For this review, take the finished solid that the model builds, in its own axes (mm). A direction names the side the tool comes from. Coordinates: 2 decimals unless noted, no trailing zeros. Write each loop counter-clockwise with the first axis right and the second up, starting at its lowest first coordinate (ties: lowest second). Pieces come first, ordered by that corner, then holes.
Autodesk Inventor part; units mm, degrees
ref_plane "YZ Plane" through (0, 0, 0) normal (1, 0, 0) x (0, 1, 0)
ref_plane "XZ Plane" through (0, 0, 0) normal (0, 1, 0) x (-1, 0, 0)
ref_plane "XY Plane" through (0, 0, 0) normal (0, 0, 1) x (1, 0, 0)
sketch "Sketch1" plane through (0, 0, 0) normal (0, 0, 1) x (1, 0, 0)
  line L0 (0, 0) -> (25.4, 0)
  line L1 (25.4, 0) -> (25.4, 25.4)
  line L2 (25.4, 25.4) -> (0, 25.4)
  line L3 (0, 25.4) -> (0, 0)
  line L4 (3.175, 22.225) -> (22.225, 22.225)
  line L5 (22.225, 22.225) -> (22.225, 3.175)
  line L6 (22.225, 3.175) -> (3.175, 3.175)
  line L7 (3.175, 3.175) -> (3.175, 22.225)
  dimension "d0" = 25.4
  dimension "d1" = 25.4
  dimension "d2" = 3.175
extrude "Extrusion1" add sketch "Sketch1" along normal blind 101.6
sketch "Sketch2" plane through (25.4, 0, 0) normal (1, 0, 0) x (0, 0, -1)
  line L0 (0, 0) -> (0, 25.4)
  line L1 (-101.6, 0) -> (-101.6, 25.4)
  line L2 (0, 0) -> (-101.6, 0)
  circle A0 centre (-88.9, 12.7) radius 2.0701
  circle A1 centre (-76.2, 12.7) radius 2.0701
  circle A2 centre (-12.7, 12.7) radius 3.3782
  dimension "d5" = 4.1402
  dimension "d6" = 12.7
  dimension "d7" = 12.7
  dimension "d10" = 12.7
  dimension "d15" = 6.7564
  dimension "d16" = 12.7
  dimension "d17" = 12.7
extrude "Extrusion2" cut sketch "Sketch2" against normal blind 101.6
properties part number "Clapper Outer Cable Hard Stop (2)"
1) The part is to be moulded in two halves that separate along Z. For faces 1 (the face through (24, 13, 0)), 2 (the face through (23.835, 10.644, 15.381)), 3 (the face through (13, 3.175, 50)), say which applies: pulls with the +Z half, pulls with the -Z half, needs draft (parallel to the pull), parting line crosses it, or undercut.
2) For L1, parallel to Y at x = 24.6, z = 76.2; L2, parallel to X at y = 11, z = 45.5 (3 decimals), list the stretches that pass through material, from the lowest coordinate up.
3) Consider section B-B (z = 56). Give the boundary of the cut face in (x, y) (3 decimals).
4) Consider section D-D (y = 12.7). Count the separate pieces of the cut face and the enclosed holes in it, then the cut area to 3 significant figures.
5) Consider section A-A (y = 5). Give the boundary of the cut face in (x, z) (3 decimals), then the cut area to 3 significant figures.
6) Tool access review of faces 4 (the face through (1.61, 10.644, 15.381)), 5 (the face through (22.225, 13, 50)): name each direction out of +Z, -Z, +X, -X, +Y, -Y from which nothing blocks a thin tool from reaching the whole face with its end or side.
7) Clearance check with a flat-ended pin moving along its axis: P1, Ø2, axis at y = 12, z = 17.5, coming from the -X side. State where the tip first meets the part, or that it passes through.
Results:
1. face 1: pulls with the -Z half
1. face 2: undercut
1. face 3: needs draft
2. L1: y = 0 to 10.63, 14.77 to 25.4
2. L2: x = 0 to 3.175, 22.225 to 25.4
3. outline: (0, 0) - (25.4, 0) - (25.4, 25.4) - (0, 25.4) - close; hole (3.175, 3.175) - (22.225, 3.175) - (22.225, 22.225) - (3.175, 22.225) - close
4. separate pieces: 8
4. enclosed holes: 0
4. area: 550 mm2
5. outline: (0, 0) - (3.175, 0) - (3.175, 101.6) - (0, 101.6) - close; (22.225, 0) - (25.4, 0) - (25.4, 101.6) - (22.225, 101.6) - close
5. area: 645 mm2
6. face 4: +X, -X
6. face 5: +Z, -Z
7. P1: stops at x = 0
